```python
from build123d import *

# Parameters (mm, degrees)
F1_R          = 5
F2_DEPTH      = 34.64052
F3_W          = 5.08
F3_H          = 2.89434
F4_DEPTH      = 34.64052
F6_W          = 2.54
F6_H          = 7.62
F7_DEPTH      = 3.81
F7_DEPTH_BACK = 3.81
F8_R          = 0.762
F9_R          = 0.508
F10_R         = 4.826
F11_DEPTH     = 2.032
F12_W         = 10.16
F12_H         = 10.16
F13_DEPTH     = 5.08
F14_R         = 3.0734
F15_DEPTH     = 5.08
F16_W         = 10.16
F16_H         = 10.16
F17_DEPTH     = 6.09474
F18_R         = 3.81
F19_DEPTH     = 8.89
F5_R          = 3.2004
F20_DEPTH     = 31.75
F21_R         = 1.27
F22_W         = 24.48052
F22_H         = 22.7021586563
F23_DEPTH     = 25.4
F24_R         = 4.1483238307
F25_DEPTH     = 2.032


with BuildPart() as f2:
    # F1 (on Front) → F2 (new body)
    with BuildSketch(Plane.XZ):
        Circle(F1_R)
    extrude(amount=-F2_DEPTH)

    # F3 (on face) → F4 (join, through all)
    with BuildSketch(Plane.XZ):
        with Locations((0, -4.64757)):
            Rectangle(F3_W, F3_H)
    extrude(amount=-F4_DEPTH)

    # F6 (on Right) → F7 (join, two sides)
    with BuildSketch(Plane.YZ) as f7_sk:
        with Locations((32.60852, 6.35)):
            Rectangle(F6_W, F6_H)
        with Locations((24.98852, 6.35)):
            Rectangle(F6_W, F6_H)
    extrude(amount=F7_DEPTH)
    extrude(f7_sk.sketch, amount=-F7_DEPTH_BACK)

    # F8
    f8_edges = [f2.edges().sort_by_distance(p)[0] for p in [
        (0, 26.25852, 10.16),
        (0, 31.33852, 10.16),
        (0, 33.87852, 10.16),
        (0, 23.71852, 10.16),
        (-3.81, 26.25852, 6.698943),
        (-3.81, 23.71852, 6.698943),
        (-3.81, 24.98852, 10.16),
        (-3.81, 31.33852, 6.698943),
        (-3.81, 32.60852, 10.16),
        (-3.81, 33.87852, 6.698943),
        (3.81, 24.98852, 10.16),
        (3.81, 26.25852, 6.698943),
        (3.81, 23.71852, 6.698943),
        (3.81, 31.33852, 6.698943),
        (3.81, 32.60852, 10.16),
        (3.81, 33.87852, 6.698943),
    ]]
    fillet(f8_edges, radius=F8_R)

    # F9
    f9_edges = [f2.edges().sort_by_distance(p)[0] for p in [
        (-2.54, 17.32026, -6.09474),
        (2.54, 17.32026, -6.09474),
    ]]
    fillet(f9_edges, radius=F9_R)

    # F10 (on face) → F11 (join)
    with BuildSketch(Plane.XZ):
        Circle(F10_R)
    extrude(amount=-F11_DEPTH)

    # F12 (on Top) → F13 (join)
    with BuildSketch(Plane.XY):
        with Locations((0, 5.08)):
            Rectangle(F12_W, F12_H)
    extrude(amount=F13_DEPTH)

    # F14 (on face) → F15 (cut)
    with BuildSketch(Plane.XY.offset(5.08)):
        with Locations((0, 5.08)):
            Circle(F14_R)
    extrude(amount=-F15_DEPTH, mode=Mode.SUBTRACT)

    # F16 (on Top) → F17 (join, through all)
    with BuildSketch(Plane.XY):
        with Locations((0, 29.56052)):
            Rectangle(F16_W, F16_H)
    extrude(amount=-F17_DEPTH)

    # F18 (on face) → F19 (cut)
    with BuildSketch(Plane(origin=(0, 0, -6.09474), x_dir=(1, 0, 0), z_dir=(0, 0, -1))):
        with Locations((0, -29.56052)):
            Circle(F18_R)
    extrude(amount=-F19_DEPTH, mode=Mode.SUBTRACT)

    # F5 (on face) → F20 (cut)
    with BuildSketch(Plane.XZ):
        Circle(F5_R)
    extrude(amount=-F20_DEPTH, mode=Mode.SUBTRACT)

    # F21
    f21_edges = [f2.edges().sort_by_distance(p)[0] for p in [
        (-2.070993, 32.758502, 2.79526),
        (3.197982, 27.489527, 2.79526),
    ]]
    fillet(f21_edges, radius=F21_R)

    # F22 (on face) → F23 (cut)
    with BuildSketch(Plane(origin=(-5.08, 0, 0), x_dir=(0, -1, 0), z_dir=(-1, 0, 0))):
        with Locations((-22.40026, 5.2563393282)):
            Rectangle(F22_W, F22_H)
    extrude(amount=-F23_DEPTH, mode=Mode.SUBTRACT)

    # F24 (on face) → F25 (join)
    with BuildSketch(Plane.XZ):
        Circle(F24_R)
    extrude(amount=-F25_DEPTH)


solid = f2.part
```
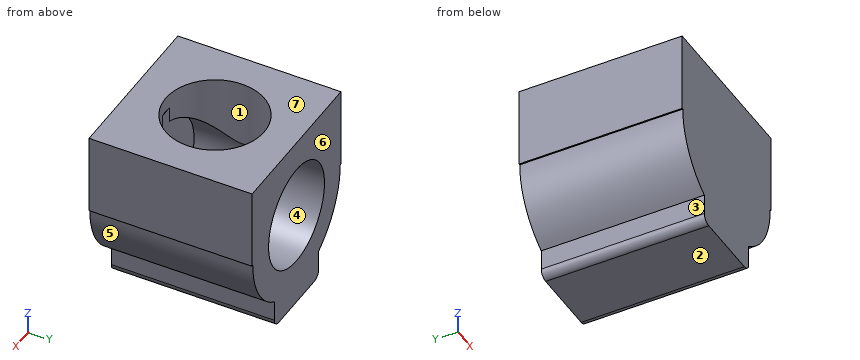
Check sheet for the modelled part. Datum: model origin and axes. Units: mm. Face numbers are marked on the shaded views. A direction names the side the tool comes from. Give positions to 0.01 mm unless a question says otherwise; leave off trailing zeros. Loops run counter-clockwise (first coordinate to the right, second up) from the corner with the lowest first, then second, coordinate; pieces in that order, holes last. Notation, with made-up numbers: M 77,82 L 129,82 A13 cw 129,101 Z; hole C 74,0 d9. An arc over 180 degrees is marked long. Answer as CSV lines item,"result".
Item 1: Sectioned sample at D-D, the plane z = 2. Enter the section's corners in (x, y), then the cut area to 3 significant figures.
Reply:
outline,"M -5.08,0 L 5.08,0 L 5.08,10.16 L 2.5,10.16 L 2.5,6.87 A3.07 cw 2.5,3.29 L 2.5,2.03 L -2.5,2.03 L -2.5,3.29 A3.07 cw -2.5,6.87 L -2.5,10.16 L -5.08,10.16 Z"
area,"59.8 mm^2"
Item 2: Sectioned sample at C-C, the plane y = 1.25. Enter the section's corners in (x, z).
Reply:
outline,"M -5.08,0 L -5,0 A5 ccw -2.54,-4.31 L -2.54,-5.59 A0.51 ccw -2.03,-6.09 L 2.03,-6.09 A0.51 ccw 2.54,-5.59 L 2.54,-4.31 A5 ccw 5,0 L 5.08,0 L 5.08,5.08 L -5.08,5.08 Z"
Item 3: Sectioned sample at A-A, the plane y = 9.25. Enter the section's corners in (x, z).
Reply:
outline,"M -5.08,0 L -5,0 A5 ccw -2.54,-4.31 L -2.54,-5.59 A0.51 ccw -2.03,-6.09 L 2.03,-6.09 A0.51 ccw 2.54,-5.59 L 2.54,-4.31 A5 ccw 5,0 L 5.08,0 L 5.08,5.08 L -5.08,5.08 Z; hole C 0,0 d6.4"
Item 4: Draft check along Z on the marked faces 4, 5, 6 and 7. Enter one of: pulls with the +Z half, pulls with the -Z half, needs draft (parallel to the pull), parting line crosses it, or undercut.
Reply:
face 4,"undercut"
face 5,"pulls with the -Z half"
face 6,"needs draft"
face 7,"pulls with the +Z half"
Item 5: Depth check by flat-ended pin: pin 1 Ø3 at (x, z) = (0.5, 0.5) entering from +Y; pin 2 Ø6 at (y, z) = (8, -4.5) entering from -X. Enter the tip coordinate at first touch or a pass-through.
Reply:
pin 1,"y = 2.03"
pin 2,"x = -4.77"
Item 6: Sectioned sample at B-B, the plane x = -0.75. Enter the section's corners in (y, z), then the cut area to 3 significant figures.
Reply:
outline,"M 0,-6.09 L 10.16,-6.09 L 10.16,-3.11 L 2.03,-3.11 L 2.03,3.11 L 2.1,3.11 L 2.1,5.08 L 0,5.08 Z; M 8.06,3.11 L 10.16,3.11 L 10.16,5.08 L 8.06,5.08 Z"
area,"51.2 mm^2"
Item 7: Set-up check for the marked faces 1, 2 and 3: record each of +Z, -Z, +X, -X, +Y, -Y from which the full face is reachable in a straight line by a thin tool's end or side.
Reply:
face 1,"+Z"
face 2,"-Z, +X, -X, +Y, -Y"
face 3,"-Z, -X, +Y, -Y"
Item 8: Scan lines: L1, parallel to X at y = 5.08, z = 3.5; L2, parallel to Y at x = 0, z = 3.9; L3, parallel to Z at x = 0, y = 6.25. Record each from-to range of solid material in increasing order.
Reply:
L1,"-5.08 to -3.07, 3.07 to 5.08"
L2,"0 to 2.03, 8.15 to 10.16"
L3,"-6.09 to -3.2"
